Geometry check sheet. Reference: the model listing, model coordinates, mm. A direction names the side the tool comes from. Round coordinates to 2 decimals unless told otherwise and drop trailing zeros. Write each loop counter-clockwise with the first axis right and the second up, starting at its lowest first coordinate (ties: lowest second). Pieces come first, ordered by that corner, then holes. Notation, with made-up numbers: M 13,70 L 69,70 A21 cw 69,86 Z; hole C -19.5,36 d6. An arc over 180 degrees is marked long. Answer in a Markdown table with one row per item. Add a question column.
from build123d import *

# Parameters (mm, degrees)
F0_W      = 127
F0_H      = 127
F1_DEPTH  = 127
F2_R      = 11.1125
F3_DEPTH  = 6.35
F4_R      = 11.1125
F5_DEPTH  = 6.35
F6_R      = 11.1125
F7_DEPTH  = 6.35
F8_R      = 11.1125
F9_DEPTH  = 6.35
F10_R     = 11.1125
F11_DEPTH = 6.35
F12_R     = 11.1125
F13_DEPTH = 6.35


with BuildPart() as f1:
    # F0 (on Top) → F1 (new body)
    with BuildSketch(Plane.XY):
        with Locations((63.5, 63.5)):
            Rectangle(F0_W, F0_H)
    extrude(amount=F1_DEPTH)

    # F2 (on face) → F3 (cut)
    with BuildSketch(Plane.XY.offset(127)):
        with Locations((63.5, 63.5)):
            Circle(F2_R)
    extrude(amount=-F3_DEPTH, mode=Mode.SUBTRACT)

    # F4 (on face) → F5 (cut)
    with BuildSketch(Plane.XZ):
        with Locations((22.225, 22.225)):
            Circle(F4_R)
        with Locations((104.775, 104.775)):
            Circle(F4_R)
    extrude(amount=-F5_DEPTH, mode=Mode.SUBTRACT)

    # F6 (on face) → F7 (cut)
    with BuildSketch(Plane.YZ.offset(127)):
        with Locations((22.225, 22.225)):
            Circle(F6_R)
        with Locations((63.5, 63.5)):
            Circle(F6_R)
        with Locations((104.775, 104.775)):
            Circle(F6_R)
    extrude(amount=-F7_DEPTH, mode=Mode.SUBTRACT)

    # F8 (on face) → F9 (cut)
    with BuildSketch(Plane(origin=(0, 127, 0), x_dir=(-1, 0, 0), z_dir=(0, 1, 0))):
        with Locations((-22.225, 104.775)):
            Circle(F8_R)
        with Locations((-104.775, 104.775)):
            Circle(F8_R)
        with Locations((-104.775, 28.230721)):
            Circle(F8_R)
        with Locations((-22.225, 22.225)):
            Circle(F8_R)
    extrude(amount=-F9_DEPTH, mode=Mode.SUBTRACT)

    # F10 (on face) → F11 (cut)
    with BuildSketch(Plane(origin=(0, 0, 0), x_dir=(1, 0, 0), z_dir=(0, 0, -1))):
        with Locations((22.225, -104.775)):
            Circle(F10_R)
        with Locations((63.5, -63.5)):
            Circle(F10_R)
        with Locations((104.775, -22.225)):
            Circle(F10_R)
        with Locations((22.225, -22.225)):
            Circle(F10_R)
        with Locations((104.775, -104.775)):
            Circle(F10_R)
    extrude(amount=-F11_DEPTH, mode=Mode.SUBTRACT)

    # F12 (on face) → F13 (cut)
    with BuildSketch(Plane(origin=(0, 0, 0), x_dir=(0, -1, 0), z_dir=(-1, 0, 0))):
        with Locations((-104.775, 104.775)):
            Circle(F12_R)
        with Locations((-104.775, 63.5)):
            Circle(F12_R)
        with Locations((-104.775, 22.225)):
            Circle(F12_R)
        with Locations((-22.225, 104.775)):
            Circle(F12_R)
        with Locations((-22.225, 63.5)):
            Circle(F12_R)
        with Locations((-22.225, 22.225)):
            Circle(F12_R)
    extrude(amount=-F13_DEPTH, mode=Mode.SUBTRACT)


solid = f1.part
Item 1: Access from +Z, -Z, +X, -X, +Y, -Y to the whole of each face (thin tool, end or side, straight path). Record for faces 1 (the flat face through (22, 120.65, 105)), 2 (the cylindrical face through (3.131, 115.877, 22.714)), 3 (the flat face through (120.65, 105, 105)), 4 (the cylindrical face through (96.585, 97.265, 3.131)).
Item 2: Section check A-A, the plane x = 63.5. Record the boundary of the cut face in (y, z).
Item 3: Scan lines: probe 1 along Y at (x, z) = (4, 63); probe 2 along Y at (x, z) = (122, 63); probe 3 along Z at (x, y) = (123.75, 63.5). Record each from-to range of solid material in increasing order. Write a range as from..to.
Item 4: Section check D-D, the plane z = 19. Record the boundary of the cut face in (x, y).
Item 5: Section check C-C, the plane y = 63.5. Record the boundary of the cut face in (x, z).
Item 6: Gauge pin test, flat ends, axial feed: pin 1 Ø4 at (y, z) = (95, 82.5) entering from -X; pin 2 Ø11 at (x, z) = (104, 104) entering from -Y; pin 3 Ø6.5 at (x, z) = (110, 30) entering from +Y; pin 4 Ø6.5 at (x, y) = (100.5, 105) entering from -Z. Record the tip position at first contact, or that the pin passes through.
Item 7: Mould release check, pull along Z, two halves, no side actions. Record for faces 5 (the flat face through (48, 64, 0)), 6 (the flat face through (22, 120.65, 22)), 7 (the flat face through (48, 64, 127)): +Z half, -Z half, draft (parallel to the pull), parting line (faces both ways), or undercut.
Item 8: Section check B-B, the plane z = 63.5. Record the boundary of the cut face in (x, y), and give its area (3 significant figures).
Result sheet:
| question | item | result |
|---|---|---|
| 1 | face 1 | +Y |
| 1 | face 2 | -X |
| 1 | face 3 | +X |
| 1 | face 4 | -Z |
| 2 | outline | M 0,0 L 52.39,0 L 52.39,6.35 L 74.61,6.35 L 74.61,0 L 127,0 L 127,127 L 74.61,127 L 74.61,120.65 L 52.39,120.65 L 52.39,127 L 0,127 Z |
| 3 | probe 1 | y = 0..11.12, 33.33..93.67, 115.88..127 |
| 3 | probe 2 | y = 0..52.4, 74.6..127 |
| 3 | probe 3 | z = 0..52.39, 74.61..127 |
| 4 | outline | M 0,0 L 11.59,0 L 11.59,6.35 L 32.86,6.35 L 32.86,0 L 127,0 L 127,11.59 L 120.65,11.59 L 120.65,32.86 L 127,32.86 L 127,127 L 110.96,127 L 110.96,120.65 L 98.59,120.65 L 98.59,127 L 32.86,127 L 32.86,120.65 L 11.59,120.65 L 11.59,127 L 0,127 L 0,115.41 L 6.35,115.41 L 6.35,94.14 L 0,94.14 L 0,32.86 L 6.35,32.86 L 6.35,11.59 L 0,11.59 Z |
| 5 | outline | M 0,0 L 52.39,0 L 52.39,6.35 L 74.61,6.35 L 74.61,0 L 127,0 L 127,52.39 L 120.65,52.39 L 120.65,74.61 L 127,74.61 L 127,127 L 74.61,127 L 74.61,120.65 L 52.39,120.65 L 52.39,127 L 0,127 Z |
| 6 | pin 1 | stops at x = 0 |
| 6 | pin 2 | stops at y = 6.35 |
| 6 | pin 3 | stops at y = 120.65 |
| 6 | pin 4 | stops at z = 6.35 |
| 7 | face 5 | -Z half |
| 7 | face 6 | undercut |
| 7 | face 7 | +Z half |
| 8 | outline | M 0,0 L 127,0 L 127,52.39 L 120.65,52.39 L 120.65,74.61 L 127,74.61 L 127,127 L 0,127 L 0,115.89 L 6.35,115.89 L 6.35,93.66 L 0,93.66 L 0,33.34 L 6.35,33.34 L 6.35,11.11 L 0,11.11 Z |
| 8 | area | 15,700 mm^2 |
